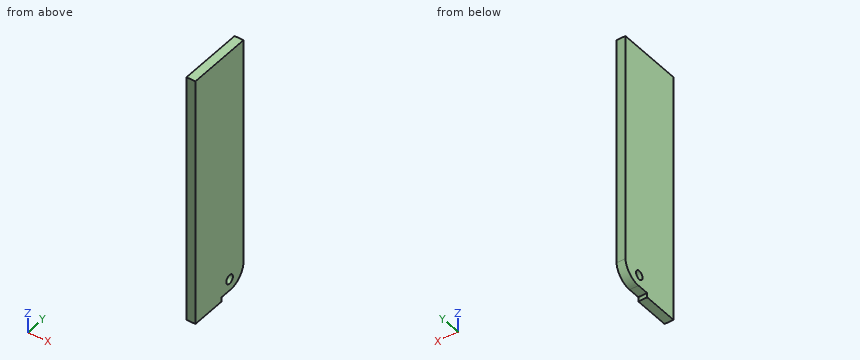
```python
from build123d import *

# Parameters (mm, degrees)
SKETCH1_R           = 1.5
BOSS_EXTRUDE1_DEPTH = 3


with BuildPart() as part:
    # Sketch1 → Boss-Extrude1 (new body)
    with BuildSketch(Plane(origin=(0, 0, 0), x_dir=(0, 0, -1), z_dir=(1, 0, 0))):
        with BuildLine():
            Line((41, 1.526420496), (42.5, 1.526420496))
            Line((42.5, 1.526420496), (42.5, -10.502465522))
            Line((42.5, -10.502465522), (-42.5, -10.502465522))
            Line((-42.5, -10.502465522), (-42.5, 11.497534478))
            Line((-42.5, 11.497534478), (35.5, 11.497534478))
            ThreePointArc((35.5, 11.497534478), (39.415467178, 9.585490654), (41, 5.526420496))
            Line((41, 5.526420496), (41, 1.526420496))
        make_face()
        with Locations((37.107006816, 5.147769804)):
            Circle(SKETCH1_R, mode=Mode.SUBTRACT)
    extrude(amount=BOSS_EXTRUDE1_DEPTH)


solid = part.part
```
Design review of the part built by this model. Coordinates are the model's own, in mm. Give positions to 0.01 mm unless a question says otherwise; leave off trailing zeros. Order: outer loops, then holes, each group sorted by start corner. A loop starts at its lowest first (then second) coordinate and runs counter-clockwise, first axis right, second up. Notation, with made-up numbers: (-7, 14) -> (9, 14) arc R19 cw to (9, 46) -> close; hole circle Ø6 at (1.5, -39). An arc over 180 degrees is marked (long way). Write item = value, one per line. Start each with the question number.
(1) We need section A-A on x = 1. Write out the cut boundary in (y, z).
(2) For pin 1 (2.5 mm diameter, centred on y = 5.15, z = -37.11, fed in from +X) (3 decimals); pin 2 (1.5 mm diameter, centred on x = 1, y = 3, fed in from -Z), all flat-tipped, find the tip position at first contact; note any pin that passes through.
(3) We need section B-B on y = 8.5. Write out the cut boundary in (x, z).
(4) To check wall thickness, follow line 1 along Z through (x, y) = (1.8, 4); line 2 along Z through (x, y) = (2.1, 3.5); line 3 along Z through (x, y) = (1.6, 7.5). State the ranges of each line that lie inside material, in increasing order.
Numbers:
q1.outline = (-10.5, -42.5) -> (1.53, -42.5) -> (1.53, -41) -> (5.53, -41) arc R5.99 ccw to (11.5, -35.5) -> (11.5, 42.5) -> (-10.5, 42.5) -> close; hole circle Ø3 at (5.15, -37.11)
q2.pin_1 = through
q2.pin_2 = -41
q3.outline = (0, -40.21) -> (3, -40.21) -> (3, 42.5) -> (0, 42.5) -> close
q4.line_1 = -41 to -38.07, -36.14 to 42.5
q4.line_2 = -41 to 42.5
q4.line_3 = -40.67 to 42.5
